Source: CAD feature listing. Evaluate the final solid. Frame: model axes, mm. Face numbers are marked on the shaded views. A direction names the side the tool comes from. Coordinates: 2 decimals unless noted, no trailing zeros. Loops run counter-clockwise (first coordinate to the right, second up) from the corner with the lowest first, then second, coordinate; pieces in that order, holes last. Notation, with made-up numbers: (19, 37.5) - (28, 37.5) arc R8 ccw to (28, 43.5) - close; hole circle Ø7 at (-36, 39.25). An arc over 180 degrees is marked (long way). Write item = value, one per line. Start each with the question number.
from build123d import *

# Parameters (mm, degrees)
F0_R     = 2.263
F1_DEPTH = 5.842


with BuildPart() as f1:
    # F0 (on Top) → F1 (new body)
    with BuildSketch(Plane.XY):
        with BuildLine():
            Line((-6.35, -14.00302), (-6.35, -19.84502))
            Line((-6.35, -19.84502), (6.35, -19.84502))
            Line((6.35, -19.84502), (6.35, -14.00302))
            Line((6.35, -14.00302), (12.7, -14.00302))
            Line((12.7, -14.00302), (5.863279, 2.438127))
            ThreePointArc((5.863279, 2.438127), (0, 6.35), (-5.863279, 2.438127))
            Line((-5.863279, 2.438127), (-12.7, -14.00302))
            Line((-12.7, -14.00302), (-6.35, -14.00302))
        make_face()
        Circle(F0_R, mode=Mode.SUBTRACT)
    extrude(amount=F1_DEPTH)


solid = f1.part
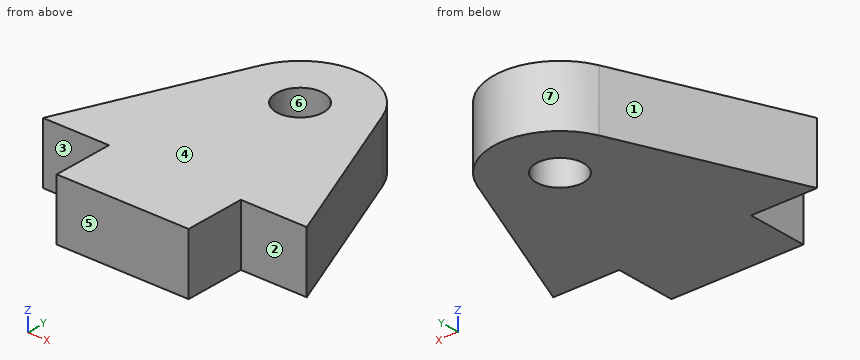
Item 1: Reachability of the marked faces 1, 2 and 3 from +Z, -Z, +X, -X, +Y, -Y: full face, straight path, thin tool, end or side. Return the list, or none.
Item 2: Cut plane D-D (y = -15.75). Return the cut outline in (x, z).
Item 3: Material intervals for L1, parallel to Y at x = 0, z = 1.8; L2, parallel to Y at x = 1.75, z = 2.75; L3, parallel to X at y = -0.75, z = 1.7, sorted ascending. Write a range as [from, to].
Item 4: Draft query along Y for the marked faces 4, 5, 6 and 7. Return one class per face: released by +Y, released by -Y, zero draft, split by the parting line, or undercut.
Item 5: Cut plane B-B (z = 4.9). Return the cut outline in (x, y), then the cut area to 3 significant figures.
Item 6: Cut plane A-A (x = 0). Return the cut outline in (y, z).
Item 7: First-contact query: pin 1 (4 mm diameter, centred on x = 9, y = -7.5, fed in from -Z); pin 2 (3 mm diameter, centred on y = -6, z = 4.5, fed in from -X); pin 3 (3 mm diameter, centred on x = 10.5, z = 4, fed in from -Y); pin 4 (1 mm diameter, centred on x = -1.5, z = 5, fed in from +Y). Flat tips, straight axial feed; report the tip coordinate or a pass-through.
Item 8: Cut plane C-C (y = 0). Return the cut outline in (x, z), then the cut area to 3 significant figures.
Responses:
q1.face_1 = +Z, -Z, -X, +Y
q1.face_2 = +Z, -Z, +X, -Y
q1.face_3 = +Z, -Z, -X, -Y
q2.outline = (-6.35, 0) - (6.35, 0) - (6.35, 5.84) - (-6.35, 5.84) - close
q3.L1 = [-19.85, -2.26], [2.26, 6.35]
q3.L2 = [-19.85, -1.43], [1.43, 6.1]
q3.L3 = [-7.19, -2.14], [2.14, 7.19]
q4.face_4 = zero draft
q4.face_5 = released by -Y
q4.face_6 = undercut
q4.face_7 = released by +Y
q5.outline = (-12.7, -14) - (-6.35, -14) - (-6.35, -19.85) - (6.35, -19.85) - (6.35, -14) - (12.7, -14) - (5.86, 2.44) arc R6.35 ccw to (-5.86, 2.44) - close; hole circle Ø4.53 at (0, 0)
q5.area = 396 mm2
q6.outline = (-19.85, 0) - (-2.26, 0) - (-2.26, 5.84) - (-19.85, 5.84) - close; (2.26, 0) - (6.35, 0) - (6.35, 5.84) - (2.26, 5.84) - close
q7.pin_1 = 0
q7.pin_2 = -10
q7.pin_3 = -14
q7.pin_4 = 6.27
q8.outline = (-6.88, 0) - (-2.26, 0) - (-2.26, 5.84) - (-6.88, 5.84) - close; (2.26, 0) - (6.88, 0) - (6.88, 5.84) - (2.26, 5.84) - close
q8.area = 53.9 mm2
